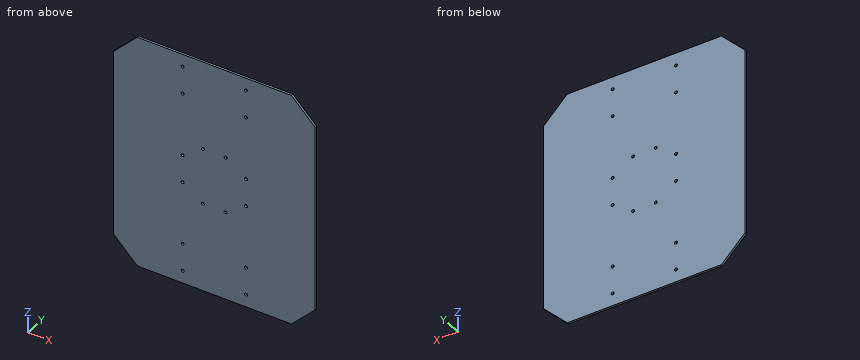
```python
from build123d import *

# Parameters (mm, degrees)
SKETCH1_R           = 2.2225
BOSS_EXTRUDE1_DEPTH = 3.175
SKETCH2_R           = 2.159
CUT_EXTRUDE1_DEPTH  = 297.247830215


with BuildPart() as part:
    # Sketch1 → Boss-Extrude1 (new body)
    with BuildSketch(Plane(origin=(0, 0, 0), x_dir=(1, 0, 0), z_dir=(0, 1, 0))):
        Polygon((-85.365028143, 123.058976948), (-121.286052627, 87.137952464), (-121.286052627, -196.619998567), (-85.365028143, -232.541023052), (147.592922888, -232.541023052), (183.513947373, -196.619998567), (183.513947373, 87.137952464), (147.592922888, 123.058976948), align=None)
        with Locations(Location((-16.765052627, -213.491023052, 0), (0, 0, 270))):
            Circle(SKETCH1_R, mode=Mode.SUBTRACT)
        with Locations(Location((-16.765052627, -171.581023052, 0), (0, 0, 270))):
            Circle(SKETCH1_R, mode=Mode.SUBTRACT)
        with Locations(Location((-16.765052627, -75.696023052, 0), (0, 0, 270))):
            Circle(SKETCH1_R, mode=Mode.SUBTRACT)
        with Locations(Location((78.992947373, -213.491023052, 0), (0, 0, 270))):
            Circle(SKETCH1_R, mode=Mode.SUBTRACT)
        with Locations(Location((78.992947373, -171.581023052, 0), (0, 0, 270))):
            Circle(SKETCH1_R, mode=Mode.SUBTRACT)
        with Locations(Location((78.992947373, -75.696023052, 0), (0, 0, 270))):
            Circle(SKETCH1_R, mode=Mode.SUBTRACT)
        with Locations(Location((-16.765052627, -33.786023052, 0), (0, 0, 270))):
            Circle(SKETCH1_R, mode=Mode.SUBTRACT)
        with Locations(Location((-16.765052627, 62.098976948, 0), (0, 0, 270))):
            Circle(SKETCH1_R, mode=Mode.SUBTRACT)
        with Locations(Location((-16.765052627, 104.008976948, 0), (0, 0, 270))):
            Circle(SKETCH1_R, mode=Mode.SUBTRACT)
        with Locations(Location((78.992947373, -33.786023052, 0), (0, 0, 270))):
            Circle(SKETCH1_R, mode=Mode.SUBTRACT)
        with Locations(Location((78.992947373, 62.098976948, 0), (0, 0, 270))):
            Circle(SKETCH1_R, mode=Mode.SUBTRACT)
        with Locations(Location((78.992947373, 104.008976948, 0), (0, 0, 270))):
            Circle(SKETCH1_R, mode=Mode.SUBTRACT)
    extrude(amount=BOSS_EXTRUDE1_DEPTH)

    # Sketch2 → Cut-Extrude1 (cut, through all)
    with BuildSketch(Plane(origin=(0, 3.175, 0), x_dir=(1, 0, 0), z_dir=(0, 1, 0))):
        with Locations(Location((13.841947373, -12.069023052, 0), (0, 0, 270))):
            Circle(SKETCH2_R)
        with Locations(Location((48.131947373, -12.069023052, 0), (0, 0, 270))):
            Circle(SKETCH2_R)
        with Locations(Location((13.841947373, -97.159023052, 0), (0, 0, 270))):
            Circle(SKETCH2_R)
        with Locations(Location((48.131947373, -97.159023052, 0), (0, 0, 270))):
            Circle(SKETCH2_R)
    extrude(amount=-CUT_EXTRUDE1_DEPTH, mode=Mode.SUBTRACT)


solid = part.part
```
Read the model definition and answer for the solid it produces. Units are mm, in the model's axes. Coordinates: 2 decimals unless noted, no trailing zeros. Write each loop counter-clockwise with the first axis right and the second up, starting at its lowest first coordinate (ties: lowest second). Pieces come first, ordered by that corner, then holes. Notation, with made-up numbers: (51.5, -16.75) -> (61.5, -16.75) arc R22 cw to (61.5, -7.75) -> close; hole circle Ø11 at (3, -36). An arc over 180 degrees is marked (long way). Answer as a JSON object with one key per item and string values.
Q1. A flat-ended cylindrical pin translates along its axis: pin 1 Ø4 at (x, z) = (-16.77, -104.01) entering from -Y. Find the tip coordinate at first contact, or state that the pin passes through.
The answers:
{"pin 1": "passes through"}
Q2. The part is cut by section A-A on y = 1.4. Give the number of separate pieces and of enclosed holes in the cut face, then the cut area to 3 significant figures.
The answers:
{"separate pieces": "1", "enclosed holes": "16", "area": "106,000 mm2"}
Q3. The part is cut by section B-B on x = 152.5. Give the vertices of the cut face in (y, z) (3 decimals).
The answers:
{"outline": "(0, -118.152) -> (3.175, -118.152) -> (3.175, 227.634) -> (0, 227.634) -> close"}
Q4. Consider line 1 (Z direction, x = 157, y = 1.5). Determine where the line is inside the solid, lowest interval first. Write a range as [from, to].
The answers:
{"line 1": "z = [-113.65, 223.13]"}
